Source: CAD feature listing. Evaluate the final solid. Frame: model axes, mm. Face numbers are marked on the shaded views. A direction names the side the tool comes from. Give positions to 0.01 mm unless a question says otherwise; leave off trailing zeros. Write each loop counter-clockwise with the first axis right and the second up, starting at its lowest first coordinate (ties: lowest second). Pieces come first, ordered by that corner, then holes. Notation, with made-up numbers: (81, 77) -> (92, 77) arc R16 cw to (92, 89) -> close; hole circle Ø5 at (3.5, -1.5). An arc over 180 degrees is marked (long way). Write item = value, one per line.
from build123d import *

# Parameters (mm, degrees)
F0_R     = 10.922
F1_DEPTH = 3.048
F2_R     = 2.54
F3_R     = 3.683
F4_DEPTH = 4.445


with BuildPart() as f1:
    # F0 (on Top) → F1 (new body)
    with BuildSketch(Plane.XY):
        Circle(F0_R)
    extrude(amount=F1_DEPTH)

    # F2
    f2_edges = [f1.edges().sort_by_distance(p)[0] for p in [
        (-10.922, 0, 0),
    ]]
    fillet(f2_edges, radius=F2_R)

    # F3 (on face) → F4 (join)
    with BuildSketch(Plane.XY.offset(3.048)):
        Circle(F3_R)
    extrude(amount=F4_DEPTH)


solid = f1.part
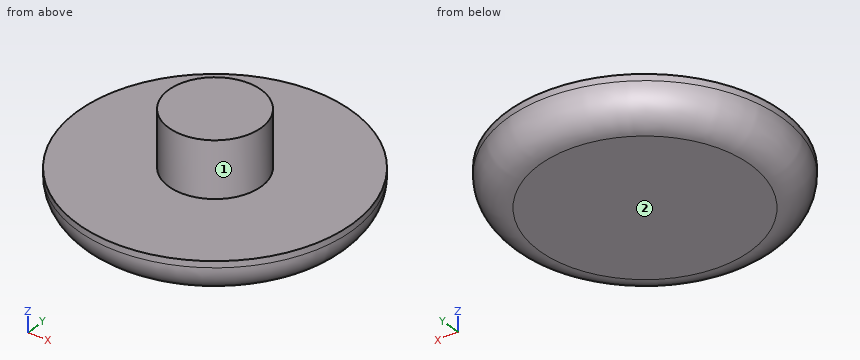
(1) First-contact query: pin 1 (2 mm diameter, centred on x = -3, y = 7.5, fed in from +Z); pin 2 (3 mm diameter, centred on y = -7, z = 2, fed in from -X); pin 3 (3 mm diameter, centred on x = -0.5, z = 5, fed in from -Y); pin 4 (11 mm diameter, centred on x = -4, y = -3, fed in from +Z). Flat tips, straight axial feed; report the tip coordinate or a pass-through.
Values follow:
pin_1 = 3.05
pin_2 = -9.41
pin_3 = -3.68
pin_4 = 7.49
(2) Section query A-A (x = 0). Return loops of the section in (y, z).
Values follow:
outline = (-10.92, 2.54) arc R2.54 ccw to (-8.38, 0) -> (8.38, 0) arc R2.54 ccw to (10.92, 2.54) -> (10.92, 3.05) -> (3.68, 3.05) -> (3.68, 7.49) -> (-3.68, 7.49) -> (-3.68, 3.05) -> (-10.92, 3.05) -> close
(3) Section query D-D (z = 1). Return loops of the section in (x, y).
Values follow:
outline = circle Ø20.8 at (0, 0)
(4) Section query C-C (z = 3.75). Return loops of the section in (x, y), plus the area to 3 significant figures.
Values follow:
outline = circle Ø7.37 at (0, 0)
area = 42.6 mm2
(5) Material intervals for line 1 (Z direction, x = -5.75, y = -5.75); line 2 (Y direction, x = -3.5, z = 2); line 3 (Y direction, x = -5, z = 2.5), sorted ascending.
Values follow:
line_1 = 0 to 3.05
line_2 = -10.28 to 10.28
line_3 = -9.71 to 9.71
(6) Access query for the marked faces 1 and 2. Directions: +Z, -Z, +X, -X, +Y, -Y. A direction counts if a zero-diameter tool reaches every point of the face in a straight line with its end or side. Return the directions, or none.
Values follow:
face_1 = +Z
face_2 = -Z, +X, -X, +Y, -Y
